from build123d import *

# Parameters (mm, degrees)
F0_R     = 9.05
F1_DEPTH = 64.8
F2_R     = 1
F3_R     = 4.5
F4_DEPTH = 0.5
F5_R     = 0.5


with BuildPart() as f1:
    # F0 (on Top) → F1 (new body)
    with BuildSketch(Plane.XY):
        Circle(F0_R)
    extrude(amount=F1_DEPTH)

    # F2
    f2_edges = [f1.edges().sort_by_distance(p)[0] for p in [
        (-9.05, 0, 0),
    ]]
    fillet(f2_edges, radius=F2_R)

    # F3 (on face) → F4 (join)
    with BuildSketch(Plane.XY.offset(64.8)):
        Circle(F3_R)
    extrude(amount=F4_DEPTH)

    # F5
    f5_edges = [f1.edges().sort_by_distance(p)[0] for p in [
        (-9.05, 0, 64.8),
    ]]
    fillet(f5_edges, radius=F5_R)


solid = f1.part
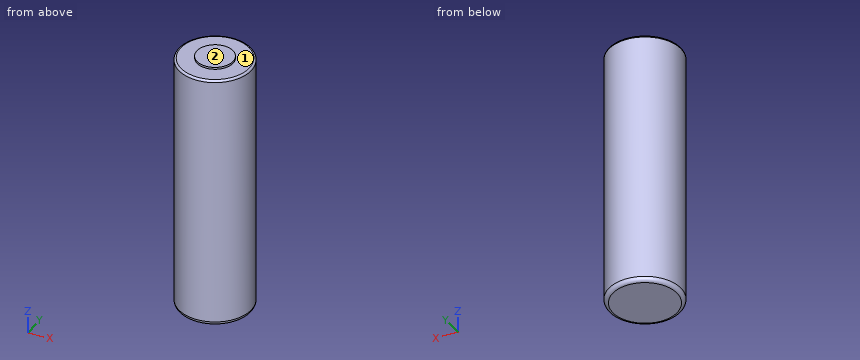
CAD build for the part. Positions are in the model's coordinates, mm. Face numbers are marked on the shaded views. A direction names the side the tool comes from. Coordinates: 2 decimals unless noted, no trailing zeros. Loops run counter-clockwise (first coordinate to the right, second up) from the corner with the lowest first, then second, coordinate; pieces in that order, holes last. Notation, with made-up numbers: (-16, -36.5) - (-3, -36.5) arc R22 ccw to (-3, -0.5) - close; hole circle Ø4 at (60, 23.25). An arc over 180 degrees is marked (long way). Use one line per item in the form item = value. Start each with the question number.
1) Band-saw the part on A-A (z = 56.5). Give the cut face in (x, y).
2) Flat gauge pins, fed straight in: pin 1 (6 mm diameter, centred on x = 3.5, z = 33, fed in from +Y); pin 2 (2 mm diameter, centred on x = 5.5, z = 58.5, fed in from +Y); pin 3 (6 mm diameter, centred on y = 5, z = 32, fed in from +X). Where does each tip first touch, or does it go through?
3) Drill centre lines: L1, parallel to Z at x = 4.5, y = 2; L2, parallel to Y at x = -0.5, z = 19.5; L3, parallel to X at y = -0.25, z = 58.5. Where is each one in solid material? Low to high. Write a range as from..to.
4) Tool access for the marked faces 1 and 2: list every direction of +Z, -Z, +X, -X, +Y, -Y with a clear straight run to the whole face (end or side of a thin tool).
Check values:
q1.outline = circle Ø18.1 at (0, 0)
q2.pin_1 = 9.04
q2.pin_2 = 7.85
q2.pin_3 = 8.83
q3.L1 = 0..64.8
q3.L2 = -9.04..9.04
q3.L3 = -9.05..9.05
q4.face_1 = +Z
q4.face_2 = +Z, +X, -X, +Y, -Y
